Could you check a few things on this drawing? It's one solid part, dimensions in mm from its lowest x, y, z. Give positions to 0.01 mm unless a question says otherwise; leave off trailing zeros. Write each loop counter-clockwise with the first axis right and the second up, starting at its lowest first coordinate (ties: lowest second). Pieces come first, ordered by that corner, then holes. Notation, with made-up numbers: M -33.5,33.5 L 7.5,33.5 A21 cw 7.5,49.5 Z; hole C 60.5,42.5 d4. An arc over 180 degrees is marked long. Answer as CSV lines item,"result". Start each with the question number.
Q1. Suppose I cut it at A-A (z = 1.15). Write out the boundary of the cut face in (x, y), then the cut area to 3 significant figures.
Q2. If I drill on line 1 along X through (y, z) = (2.5, 1.8); line 2 along Z through (x, y) = (4.8, 3), over which ranges is the centre line in solid material (lowest first)?
Q3. Thinking about a two-plate mould opening in X: for the marked faces 1, 2, 3 and 4, which applies, +X half, -X half, draft (parallel to the pull), parting line (faces both ways), or undercut?
Q4. Suppose I cut it at B-B (y = 8.5). Write out the boundary of the cut face in (x, z).
Q5. Suppose I cut it at C-C (x = 2.8). Write out the boundary of the cut face in (y, z).
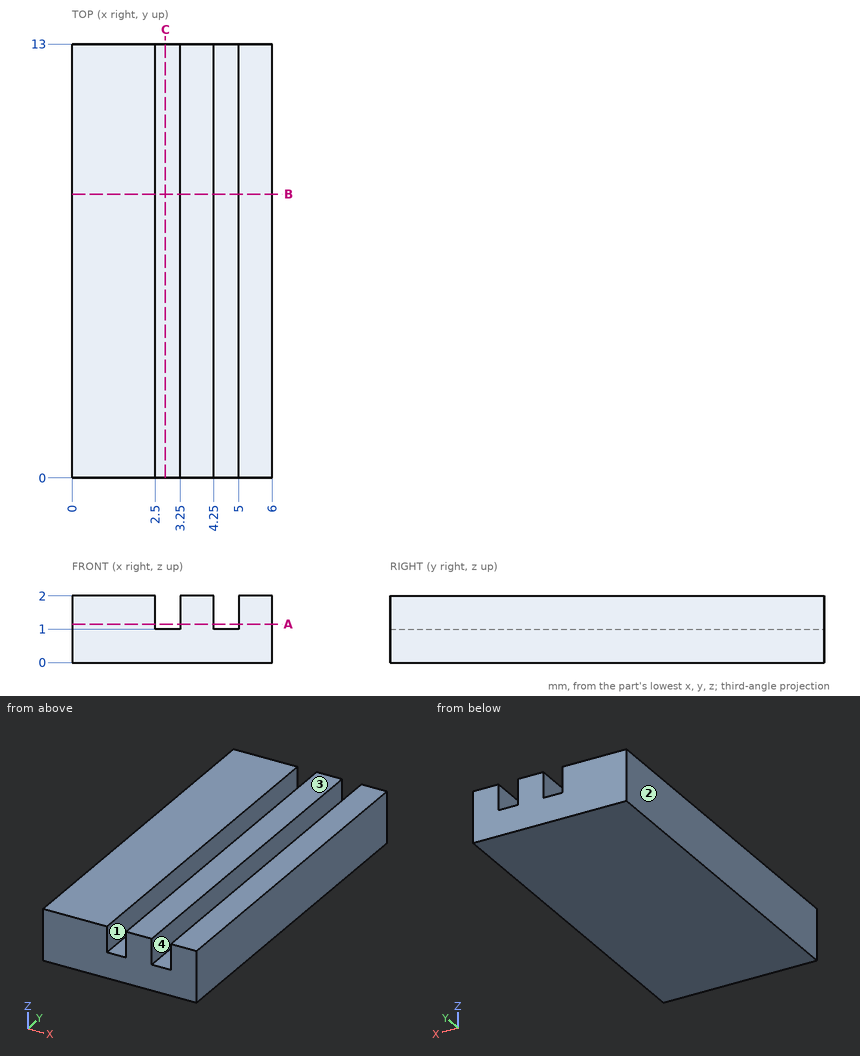
Resolved:
1,outline,"M 0,0 L 2.5,0 L 2.5,13 L 0,13 Z; M 3.25,0 L 4.25,0 L 4.25,13 L 3.25,13 Z; M 5,0 L 6,0 L 6,13 L 5,13 Z"
1,area,"58.5 mm^2"
2,line 1,"0 to 2.5, 3.25 to 4.25, 5 to 6"
2,line 2,"0 to 1"
3,face 1,"undercut"
3,face 2,"-X half"
3,face 3,"draft"
3,face 4,"undercut"
4,outline,"M 0,0 L 6,0 L 6,2 L 5,2 L 5,1 L 4.25,1 L 4.25,2 L 3.25,2 L 3.25,1 L 2.5,1 L 2.5,2 L 0,2 Z"
5,outline,"M 0,0 L 13,0 L 13,1 L 0,1 Z"
